The listing builds one solid part. Answer for the finished solid, in the listing's coordinates (mm). A direction names the side the tool comes from. Give positions to 0.01 mm unless a question says otherwise; leave off trailing zeros. Write each loop counter-clockwise with the first axis right and the second up, starting at its lowest first coordinate (ties: lowest second). Pieces come first, ordered by that corner, then holes. Notation, with made-up numbers: (42, -39.75) - (64, -39.75) arc R13 ccw to (64, -16.75) - close; hole circle Ø1 at (29.25, 29.5). An arc over 180 degrees is marked (long way). Use a Markdown table: item, result. Add a question column.
from build123d import *

# Parameters (mm, degrees)
F0_R      = 8.9789
F1_DEPTH  = 12.7
F3_R      = 5.7785
F4_DEPTH  = 9.525
F1_FACE_R = 8.9789
F4_FACE_R = 5.7785
F6_T      = -1.016


with BuildPart() as f1:
    # F0 (on Right) → F1 (new body)
    with BuildSketch(Plane.YZ):
        Circle(F0_R)
    extrude(amount=-F1_DEPTH)



with BuildPart() as f4:
    # F3 (on offset) → F4 (new body)
    with BuildSketch(Plane.YZ.offset(3.81)):
        Circle(F3_R)
    extrude(amount=F4_DEPTH)


with BuildPart() as f1_1:
    add(f1.part)

    add(f4.part)  # F5 merges F4
    # F1_face (on face) → F5 section 0
    with BuildSketch(Plane.YZ):
        Circle(F1_FACE_R)
    # F4_face (on face) → F5 section 1
    with BuildSketch(Plane(origin=(3.81, 0, 0), x_dir=(0, 1, 0), z_dir=(-1, 0, 0))):
        Circle(F4_FACE_R)
    loft()

    # F6
    f6_openings = [f1_1.faces().sort_by_distance(p)[0] for p in [
        (13.335, 0, 0),
        (-12.7, 0, 0),
    ]]
    offset(amount=F6_T, openings=f6_openings, kind=Kind.INTERSECTION)


solid = f1_1.part
1. The part is cut by section B-B (x = 8.75). Give the vertices of the cut face in (y, z) (1 decimal).
2. The part is cut by section A-A (y = 0). Give the vertices of the cut face in (x, z) (1 decimal), and give its area (3 significant figures).
3. Consider L1, parallel to Z at x = -3.75, y = 0; L2, parallel to Z at x = 11, y = 0; L3, parallel to Y at x = 1.75, z = -0.75. Determine where each line is inside the solid, lowest interval first. Write a range as [from, to].
4. For a pull along Y with two mould halves and no side action, classify faces 4 (the flat face through (13.335, 1, 5)), 5 (the conical face through (3.63, 2.74, -5.26)), 6 (the conical face through (3.255, 2.269, -4.363)) as released by +Y, released by -Y, zero draft, split by the parting line, or undercut.
5. Given P1, Ø3, axis at x = -6.5, z = -7, coming from the -Y side; P2, Ø5.5, axis at y = 0, z = 0, coming from the +X side; P3, Ø5, axis at x = -2.5, z = -2.5, coming from the -Y side; P4, Ø8, axis at x = -0.5, y = 6, coming from the +Z side, each flat-ended and moving along its own axis, determine where each tip first touches the part or whether it passes through.
6. Which of the six approach directions +Z, -Z, +X, -X, +Y, -Y give full straight-line access (tool end or side, diameter ignored) to faces 1 (the cylindrical face through (-6.261, 8.564, 2.697)), 2 (the cylindrical face through (-6.449, 7.356, -3.05)), 3 (the cylindrical face through (8.51, 3.11, 4.87))?
Check values:
| question | item | result |
|---|---|---|
| 1 | outline | circle Ø11.6 at (0, 0); hole circle Ø9.5 at (0, 0) |
| 2 | outline | (-12.7, -9) - (0, -9) - (3.8, -5.8) - (13.3, -5.8) - (13.3, -4.8) - (3.4, -4.8) - (-0.4, -8) - (-12.7, -8) - close; (-12.7, 8) - (-0.4, 8) - (3.4, 4.8) - (13.3, 4.8) - (13.3, 5.8) - (3.8, 5.8) - (0, 9) - (-12.7, 9) - close |
| 2 | area | 55.3 mm2 |
| 3 | L1 | z = [-8.98, -7.96], [7.96, 8.98] |
| 3 | L2 | z = [-5.78, -4.76], [4.76, 5.78] |
| 3 | L3 | y = [-7.47, -6.14], [6.14, 7.47] |
| 4 | face 4 | zero draft |
| 4 | face 5 | split by the parting line |
| 4 | face 6 | undercut |
| 5 | P1 | stops at y = -7.1 |
| 5 | P2 | passes through |
| 5 | P3 | stops at y = -8.98 |
| 5 | P4 | stops at z = 8.75 |
| 6 | face 1 | +X, -X |
| 6 | face 2 | -X |
| 6 | face 3 | +X |
